Can you work these out from the drawing? Everything is in mm from the part's minimum corner. Round coordinates to 2 decimals unless told otherwise and drop trailing zeros. Loops run counter-clockwise (first coordinate to the right, second up) from the corner with the lowest first, then second, coordinate; pieces in that order, holes last. Notation, with made-up numbers: (45.5, 86.5) -> (95.5, 86.5) arc R30 ccw to (95.5, 112.5) -> close; hole circle Ø6 at (-3.5, -31.75). An arc over 180 degrees is marked (long way). One line per item, written item: value.
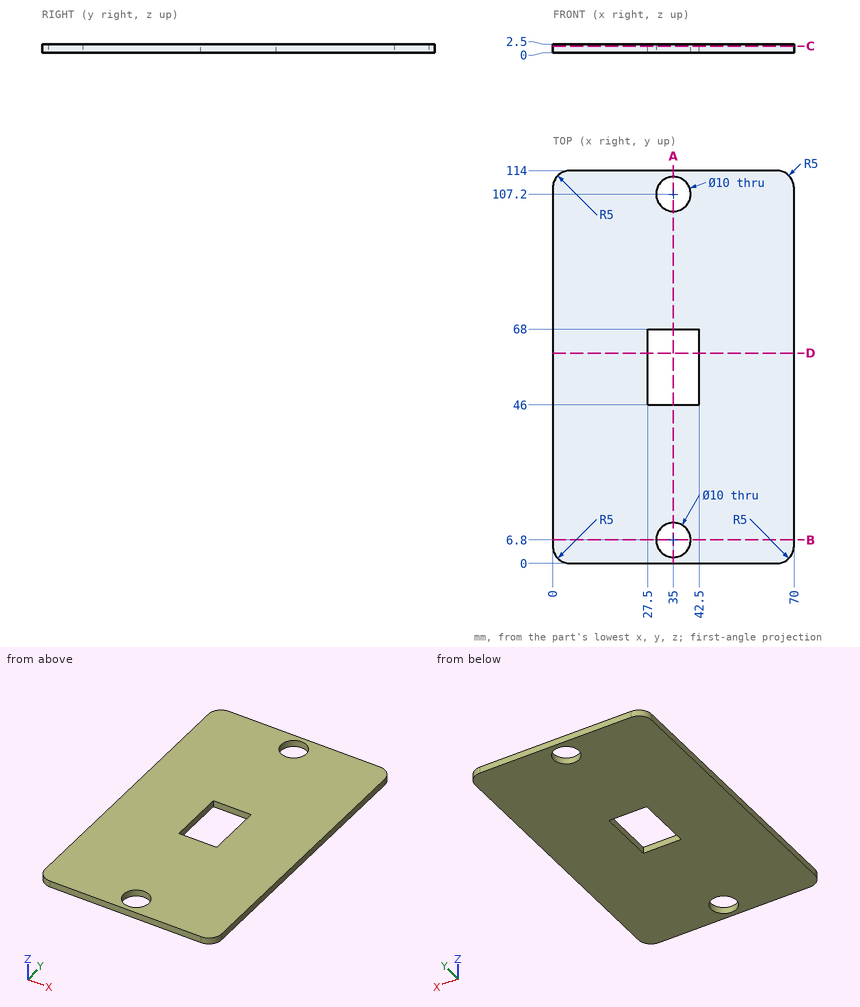
Item 1: If we section it at D-D on y = 61: List the corners of the cut face in (x, z) for me, plus the area to 4 significant figures.
Output:
outline: (0, 0) -> (27.5, 0) -> (27.5, 2.5) -> (0, 2.5) -> close; (42.5, 0) -> (70, 0) -> (70, 2.5) -> (42.5, 2.5) -> close
area: 137.5 mm²
Item 2: Will these pins go through, and if not, where does the flat tip stop? pin 1 Ø4 at (x, y) = (44.5, 59.5) entering from -Z; pin 2 Ø6 at (x, y) = (35, 107.2) entering from -Z.
Output:
pin 1: stops at z = 0
pin 2: passes through
Item 3: If we section it at B-B on y = 6.8: List the corners of the cut face in (x, z) for me.
Output:
outline: (0, 0) -> (30, 0) -> (30, 2.5) -> (0, 2.5) -> close; (40, 0) -> (70, 0) -> (70, 2.5) -> (40, 2.5) -> close
Item 4: I need wall thicknesses on line 1 (Y direction, x = 35, z = 1.4); line 2 (X direction, y = 53, z = 1.9); line 3 (Y direction, x = 39, z = 0.9). Which ranges of each line are inside material? Lowest first, please. Write a range as from..to.
Output:
line 1: y = 0..1.8, 11.8..46, 68..102.2, 112.2..114
line 2: x = 0..27.5, 42.5..70
line 3: y = 0..3.8, 9.8..46, 68..104.2, 110.2..114
Item 5: If we section it at C-C on z = 1.85: List the corners of the cut face in (x, y) for me.
Output:
outline: (0, 5) arc R5 ccw to (5, 0) -> (65, 0) arc R5 ccw to (70, 5) -> (70, 109) arc R5 ccw to (65, 114) -> (5, 114) arc R5 ccw to (0, 109) -> close; hole (27.5, 46) -> (42.5, 46) -> (42.5, 68) -> (27.5, 68) -> close; hole circle Ø10 at (35, 6.8); hole circle Ø10 at (35, 107.2)
Item 6: If we section it at A-A on x = 35: List the corners of the cut face in (y, z) for me.
Output:
outline: (0, 0) -> (1.8, 0) -> (1.8, 2.5) -> (0, 2.5) -> close; (11.8, 0) -> (46, 0) -> (46, 2.5) -> (11.8, 2.5) -> close; (68, 0) -> (102.2, 0) -> (102.2, 2.5) -> (68, 2.5) -> close; (112.2, 0) -> (114, 0) -> (114, 2.5) -> (112.2, 2.5) -> close
